```python
from build123d import *

# Parameters (mm, degrees)
SKETCH1_W           = 160
SKETCH1_H           = 77
BOSS_EXTRUDE1_DEPTH = 5
BOSS_EXTRUDE2_DEPTH = 25
SKETCH3_R           = 1.499999813
SKETCH3_R_2         = 1.5
BOSS_EXTRUDE3_DEPTH = 30
SKETCH5_W           = 39.3418497
SKETCH5_H           = 77
SKETCH5_R           = 2.947381685
BOSS_EXTRUDE5_DEPTH = 4
BOSS_EXTRUDE6_DEPTH = 5
SKETCH9_W           = 112.573012358
SKETCH9_H           = 2
BOSS_EXTRUDE7_DEPTH = 25
CUT_EXTRUDE2_START  = -74
SKETCH7_W           = 13
SKETCH7_H           = 8
CUT_EXTRUDE2_DEPTH  = 119
SKETCH6_W           = 20
SKETCH6_H           = 2
CUT_EXTRUDE1_DEPTH  = 179
SKETCH10_W          = 4
SKETCH10_H          = 3
CUT_EXTRUDE3_DEPTH  = 7
SKETCH11_W          = 105.740519207
SKETCH11_H          = 2
BOSS_EXTRUDE8_DEPTH = 8.609255


with BuildPart() as part:
    # Sketch1 → Boss-Extrude1 (new body)
    with BuildSketch(Plane(origin=(0, 0, 0), x_dir=(1, 0, 0), z_dir=(0, 1, 0))):
        with Locations((-80, -38.5)):
            Rectangle(SKETCH1_W, SKETCH1_H)
    extrude(amount=BOSS_EXTRUDE1_DEPTH)

    # Sketch2 → Boss-Extrude2 (add)
    with BuildSketch(Plane(origin=(0, 5, 0), x_dir=(1, 0, 0), z_dir=(0, 1, 0))):
        Polygon((-160, 0), (-157, 0), (-157, -74), (-3, -74), (-3, -3), (-47.4, -3), (-47.4, 0), (0, 0), (0, -77), (-160, -77), align=None)
    extrude(amount=BOSS_EXTRUDE2_DEPTH)

    # Sketch3 → Boss-Extrude3 (add)
    with BuildSketch(Plane.XZ):
        with BuildLine():
            Line((-160, 77), (-152.006026471, 77))
            Line((-152.006026471, 77), (-152.006026471, 80.326705))
            ThreePointArc((-152.006026471, 80.326705), (-156.003013236, 84.323691764), (-160, 80.326705))
            Line((-160, 80.326705), (-160, 77))
        make_face()
        with Locations((-156.003013236, 80.326705)):
            Circle(SKETCH3_R, mode=Mode.SUBTRACT)
        with BuildLine():
            Line((-47.333694812, 80.326705), (-47.333694812, 77))
            Line((-47.333694812, 77), (-39.3418497, 77))
            Line((-39.3418497, 77), (-39.3418497, 80.326705))
            ThreePointArc((-39.3418497, 80.326705), (-43.337772256, 84.322627556), (-47.333694812, 80.326705))
        make_face()
        with Locations((-43.337772256, 80.326705)):
            Circle(SKETCH3_R_2, mode=Mode.SUBTRACT)
        with BuildLine():
            Line((-160, 0), (-152.006026471, 0))
            Line((-152.006026471, 0), (-152.006026471, -3.613332))
            ThreePointArc((-152.006026471, -3.613332), (-156.003013236, -7.610318764), (-160, -3.613332))
            Line((-160, -3.613332), (-160, 0))
        make_face()
        with Locations((-156.003013236, -3.613332)):
            Circle(SKETCH3_R_2, mode=Mode.SUBTRACT)
        with BuildLine():
            Line((-47.333694812, -3.613332), (-47.333694812, 0))
            Line((-47.333694812, 0), (-39.3418497, 0))
            Line((-39.3418497, 0), (-39.3418497, -3.613332))
            ThreePointArc((-39.3418497, -3.613332), (-43.337772256, -7.609254556), (-47.333694812, -3.613332))
        make_face()
        with Locations((-43.337772256, -3.613332)):
            Circle(SKETCH3_R_2, mode=Mode.SUBTRACT)
    extrude(amount=-BOSS_EXTRUDE3_DEPTH)

    # Sketch5 → Boss-Extrude5 (add)
    with BuildSketch(Plane(origin=(0, 30, 0), x_dir=(1, 0, 0), z_dir=(0, 1, 0))):
        with Locations((-19.67092485, -38.5)):
            Rectangle(SKETCH5_W, SKETCH5_H)
        with Locations((-9.3881, -11.3566)):
            Circle(SKETCH5_R, mode=Mode.SUBTRACT)
    extrude(amount=BOSS_EXTRUDE5_DEPTH)

    # Sketch8 → Boss-Extrude6 (add)
    with BuildSketch(Plane.XZ):
        with BuildLine():
            ThreePointArc((-152.006026471, -3.613332), (-153.144295011, -6.4068304), (-155.910784614, -7.609254556))
            Line((-155.910784614, -7.609254556), (-43.337772256, -7.609254556))
            ThreePointArc((-43.337772256, -7.609254556), (-46.163316193, -6.438875937), (-47.333694812, -3.613332))
            Line((-47.333694812, -3.613332), (-47.333694812, 0))
            Line((-47.333694812, 0), (-152.006026471, 0))
            Line((-152.006026471, 0), (-152.006026471, -3.613332))
        make_face()
    extrude(amount=-BOSS_EXTRUDE6_DEPTH)

    # Sketch9 → Boss-Extrude7 (add)
    with BuildSketch(Plane(origin=(0, 5, 0), x_dir=(1, 0, 0), z_dir=(0, 1, 0))):
        with Locations((-99.624278435, 6.609254556)):
            Rectangle(SKETCH9_W, SKETCH9_H)
    extrude(amount=BOSS_EXTRUDE7_DEPTH)

    # Sketch7 → Cut-Extrude2 (cut)
    with BuildSketch(Plane(origin=(0, 0, 0), x_dir=(-1, 0, 0), z_dir=(0, 0, -1)).offset(CUT_EXTRUDE2_START)):
        with Locations((145.6418497, 9)):
            Rectangle(SKETCH7_W, SKETCH7_H)
    extrude(amount=-CUT_EXTRUDE2_DEPTH, mode=Mode.SUBTRACT)

    # Sketch6 → Cut-Extrude1 (cut)
    with BuildSketch(Plane.XY.offset(77)):
        with Locations((-135, 6)):
            Rectangle(SKETCH6_W, SKETCH6_H)
        with Locations((-65, 6)):
            Rectangle(SKETCH6_W, SKETCH6_H)
    extrude(amount=-CUT_EXTRUDE1_DEPTH, mode=Mode.SUBTRACT)

    # Sketch10 → Cut-Extrude3 (cut)
    with BuildSketch(Plane(origin=(0, 30, 0), x_dir=(1, 0, 0), z_dir=(0, 1, 0))):
        with Locations((-41.4918497, -75.5)):
            Rectangle(SKETCH10_W, SKETCH10_H)
    extrude(amount=-CUT_EXTRUDE3_DEPTH, mode=Mode.SUBTRACT)

    # Sketch11 → Boss-Extrude8 (add)
    with BuildSketch(Plane.XY.offset(-5.609254556)):
        with Locations((-99.669778561, 29)):
            Rectangle(SKETCH11_W, SKETCH11_H)
    extrude(amount=BOSS_EXTRUDE8_DEPTH)


solid = part.part
```
Design review of the part built by this model. Coordinates are the model's own, in mm. A direction names the side the tool comes from. Coordinates: 2 decimals unless noted, no trailing zeros. Order: outer loops, then holes, each group sorted by start corner. A loop starts at its lowest first (then second) coordinate and runs counter-clockwise, first axis right, second up. Notation, with made-up numbers: M 83,74 L 100,74 A15 cw 100,87 Z; hole C -33,39.25 d6. An arc over 180 degrees is marked long. Answer as a JSON object with one key per item and string values. Group by question number.
1) Tool access review of faces 4 (the flat face through (-152.006, 2, 79)), 5 (the flat face through (-139.142, 10, 75)), 6 (the flat face through (-47.4, 16, 2)), 7 (the flat face through (-39.492, 27, 76)), 8 (the flat face through (-39.342, 15, 79)): name each direction out of +Z, -Z, +X, -X, +Y, -Y from which nothing blocks a thin tool from reaching the whole face with its end or side.
2) Add section A-A, the plane x = -134.5. Write out the cut boundary in (y, z).
3) Wall thickness on L1, parallel to Z at x = -136.5, y = 21; L2, parallel to X at y = 13.5, z = 37; L3, parallel to Z at x = -7, y = 18: over which ranges is each line inside the solid? List them lowest first.
4) Add section C-C, the plane x = -19. Write out the cut boundary in (y, z), then the cut area to 3 significant figures.
5) Mouldability with a two-part tool opening along Y and no side actions: class faces 1 (the flat face through (-20, 34, 38)), 2 (the cylindrical face through (-158.764, 14.79, -6.503)), 3 (the flat face through (-100, 16, -5.609)) as pulls with the +Y half, pulls with the -Y half, needs draft (parallel to the pull), parting line crosses it, or undercut.
6) For pin 1 (1.6 mm diameter, centred on y = 6.5, z = -6.5, fed in from -X); pin 2 (8 mm diameter, centred on x = -23, z = 50.5, fed in from -Y); pin 3 (6 mm diameter, centred on x = -59, z = 68.5, fed in from +Y); pin 4 (1 mm diameter, centred on y = 12.5, z = 79, fed in from +X), all flat-tipped, find the tip position at first contact; note any pin that passes through.
7) Add section B-B, the plane y = 25.5. Count the separate pieces of the cut face and the enclosed holes in it, then the cut area to 3 significant figures.
Computed values:
{
 "1": {"face 4": "+Z, +Y, -Y", "face 5": "+Z", "face 6": "none", "face 7": "+Y", "face 8": "+Z, +X, +Y, -Y"},
 "2": {"outline": "M 0,-7.61 L 5,-7.61 L 5,77 L 0,77 Z; M 7,-7.61 L 30,-7.61 L 30,3 L 28,3 L 28,-5.61 L 7,-5.61 Z; M 7,74 L 30,74 L 30,77 L 7,77 Z"},
 "3": {"L1": "z = -7.61 to -5.61, 74 to 77", "L2": "x = -160 to -157, -3 to 0", "L3": "z = 0 to 3, 74 to 77"},
 "4": {"outline": "M 0,0 L 34,0 L 34,77 L 0,77 Z; hole M 5,3 L 30,3 L 30,74 L 5,74 Z", "area": "843 mm^2"},
 "5": {"face 1": "pulls with the +Y half", "face 2": "needs draft", "face 3": "undercut"},
 "6": {"pin 1": "stops at x = -159.41", "pin 2": "stops at y = 0", "pin 3": "stops at y = 5", "pin 4": "stops at x = -39.34"},
 "7": {"separate pieces": "1", "enclosed holes": "5", "area": "1,440 mm^2"}
}
